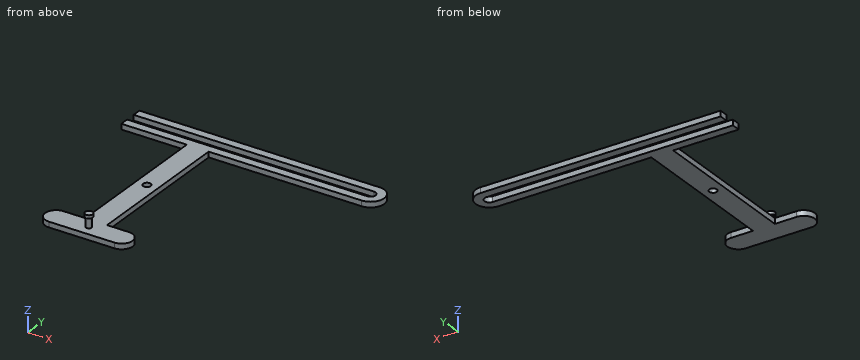
from build123d import *

# Parameters (mm, degrees)
BOSS_EXTRUDE1_DEPTH = 3.175
SKETCH4_W           = 25.4
SKETCH4_H           = 177.8
BOSS_EXTRUDE2_DEPTH = 3.175
BOSS_EXTRUDE3_DEPTH = 3.175
CUT_EXTRUDE1_DEPTH  = 304.357916701
SKETCH7_R           = 4.445
CUT_EXTRUDE2_DEPTH  = 304.357916701
SKETCH9_R           = 3.175
BOSS_EXTRUDE6_DEPTH = 15.24
SKETCH10_R          = 4.445
BOSS_EXTRUDE7_DEPTH = 3.81


with BuildPart() as part:
    # Sketch3 → Boss-Extrude1 (new, symmetric)
    with BuildSketch(Plane.XY):
        with BuildLine():
            Line((-38.1, 12.7), (38.1, 12.7))
            ThreePointArc((38.1, 12.7), (50.8, 0), (38.1, -12.7))
            Line((38.1, -12.7), (-38.1, -12.7))
            ThreePointArc((-38.1, -12.7), (-50.8, 0), (-38.1, 12.7))
        make_face()
    extrude(amount=BOSS_EXTRUDE1_DEPTH, both=True)

    # Sketch4 → Boss-Extrude2 (add, symmetric)
    with BuildSketch(Plane.XY):
        with Locations((0, 101.6)):
            Rectangle(SKETCH4_W, SKETCH4_H)
    extrude(amount=BOSS_EXTRUDE2_DEPTH, both=True)

    # Sketch5 → Boss-Extrude3 (add, symmetric)
    with BuildSketch(Plane.XY):
        with BuildLine():
            Line((-88.9, 222.25), (190.5, 222.25))
            ThreePointArc((190.5, 222.25), (206.375, 206.375), (190.5, 190.5))
            Line((190.5, 190.5), (-88.9, 190.5))
            Line((-88.9, 190.5), (-88.9, 222.25))
        make_face()
    extrude(amount=BOSS_EXTRUDE3_DEPTH, both=True)

    # Sketch6 → Cut-Extrude1 (cut, through all)
    with BuildSketch(Plane.XY.offset(3.175)):
        with BuildLine():
            Line((-88.9, 212.09), (-88.9, 200.66))
            Line((-88.9, 200.66), (190.5, 200.66))
            ThreePointArc((190.5, 200.66), (196.215, 206.375), (190.5, 212.09))
            Line((190.5, 212.09), (-88.9, 212.09))
        make_face()
    extrude(amount=-CUT_EXTRUDE1_DEPTH, mode=Mode.SUBTRACT)

    # Sketch7 → Cut-Extrude2 (cut, through all)
    with BuildSketch(Plane.XY.offset(3.175)):
        with Locations((0, 101.6)):
            Circle(SKETCH7_R)
    extrude(amount=-CUT_EXTRUDE2_DEPTH, mode=Mode.SUBTRACT)

    # Sketch9 → Boss-Extrude6 (add)
    with BuildSketch(Plane.XY.offset(3.175)):
        with Locations(Location((0, 0, 0), (0, 0, 180))):
            Circle(SKETCH9_R)
    extrude(amount=BOSS_EXTRUDE6_DEPTH)

    # Sketch10 → Boss-Extrude7 (add)
    with BuildSketch(Plane.XY.offset(18.415)):
        Circle(SKETCH10_R)
    extrude(amount=-BOSS_EXTRUDE7_DEPTH)


solid = part.part
Verification items for the finished model (mm, model axes). Round coordinates to 2 decimals unless told otherwise and drop trailing zeros. Loops run counter-clockwise (first coordinate to the right, second up) from the corner with the lowest first, then second, coordinate; pieces in that order, holes last. Notation, with made-up numbers: (71.25, -11) - (81.25, -11) arc R17 cw to (81.25, -6) - close; hole circle Ø9 at (83, 17). An arc over 180 degrees is marked (long way). Write item = value, one per line.
Q1. Sectioned sample at C-C on y = 0. Record the boundary of the cut face in (x, z) (3 decimals), plus the area to 3 significant figures.
Here are the results:
outline = (-50.8, -3.175) - (50.8, -3.175) - (50.8, 3.175) - (3.175, 3.175) - (3.175, 14.605) - (4.445, 14.605) - (4.445, 18.415) - (-4.445, 18.415) - (-4.445, 14.605) - (-3.175, 14.605) - (-3.175, 3.175) - (-50.8, 3.175) - close
area = 752 mm^2
Q2. Sectioned sample at B-B on y = 101.6. Record the boundary of the cut face in (x, z) (3 decimals), plus the area to 3 significant figures.
Here are the results:
outline = (-12.7, -3.175) - (-4.445, -3.175) - (-4.445, 3.175) - (-12.7, 3.175) - close; (4.445, -3.175) - (12.7, -3.175) - (12.7, 3.175) - (4.445, 3.175) - close
area = 105 mm^2
Q3. Material ranges on L1, parallel to Y at x = 0, z = 1 (3 decimals); L2, parallel to Y at x = 27.5, z = 2; L3, parallel to Y at x = 52, z = -0.75, recorded low to high.
Here are the results:
L1 = -12.7 to 97.155, 106.045 to 200.66, 212.09 to 222.25
L2 = -12.7 to 12.7, 190.5 to 200.66, 212.09 to 222.25
L3 = 190.5 to 200.66, 212.09 to 222.25
Q4. Depth check by flat-ended pin: pin 1 (1.9 mm diameter, centred on x = 62, z = -1, fed in from -Y); pin 2 (5 mm diameter, centred on y = 85.5, z = 1.5, fed in from +X); pin 3 (8 mm diameter, centred on x = -37, z = 3.5, fed in from +Y); pin 4 (1.9 mm diameter, centred on y = 79.5, z = -0.5, fed in from -X). Enter the tip coordinate at first touch or a pass-through.
Here are the results:
pin_1 = 190.5
pin_2 = 12.7
pin_3 = 222.25
pin_4 = -12.7
Q5. Sectioned sample at D-D on z = 8.25. Record the boundary of the cut face in (x, y) (3 decimals), plus the area to 3 significant figures.
Here are the results:
outline = circle Ø6.35 at (0, 0)
area = 31.7 mm^2
Q6. Sectioned sample at A-A on x = 9. Record the boundary of the cut face in (y, z) (3 decimals), plus the area to 3 significant figures.
Here are the results:
outline = (-12.7, -3.175) - (200.66, -3.175) - (200.66, 3.175) - (-12.7, 3.175) - close; (212.09, -3.175) - (222.25, -3.175) - (222.25, 3.175) - (212.09, 3.175) - close
area = 1,420 mm^2
